from build123d import *

# Parameters (mm, degrees)
SKETCH1_R           = 9.5
BOSS_EXTRUDE1_DEPTH = 35
CUT_EXTRUDE1_DEPTH  = 4


with BuildPart() as part:
    # Sketch1 → Boss-Extrude1 (new body)
    with BuildSketch(Plane.XY):
        Circle(SKETCH1_R)
    extrude(amount=BOSS_EXTRUDE1_DEPTH)

    # Sketch4 → Cut-Extrude1 (cut)
    with BuildSketch(Plane(origin=(0, 10, 0), x_dir=(1, 0, 0), z_dir=(0, 1, 0))):
        with BuildLine():
            Line((3, 0), (3, -25))
            ThreePointArc((3, -25), (0, -28), (-3, -25))
            Line((-3, -25), (-3, 0))
            Line((-3, 0), (3, 0))
        make_face()
    extrude(amount=-CUT_EXTRUDE1_DEPTH, mode=Mode.SUBTRACT)


solid = part.part
Source: CAD feature listing. Evaluate the final solid. Frame: model axes, mm. A direction names the side the tool comes from. Give positions to 0.01 mm unless a question says otherwise; leave off trailing zeros. Write each loop counter-clockwise with the first axis right and the second up, starting at its lowest first coordinate (ties: lowest second). Pieces come first, ordered by that corner, then holes. Notation, with made-up numbers: M 73,-5.5 L 104,-5.5 A11 cw 104,4.5 Z; hole C 3,15 d7. An arc over 180 degrees is marked long. Return JSON: item names as keys, results as strings. Group by question number.
1) Set-up query: faces 1 (the face through (-3, 8, 13)), 2 (the face through (0, 0, 35)). Return all of +Z, -Z, +X, -X, +Y, -Y with unobstructed straight access to the full face (end or side cutting, diameter ignored); none if empty.
2) Cut plane A-A, the plane x = 0. Output: boundary loops of the cut face in (y, z), then the cut area to 3 significant figures.
3) Cut plane C-C, the plane y = -2.5. Output: boundary loops of the cut face in (x, z).
4) Ray query, L1, parallel to Y at x = -0.25, z = 30.5; L2, parallel to Y at x = 7, z = 17.5; L3, parallel to X at y = -2.75, z = 15.5. Return the intervals inside material, ascending.
5) Cut plane B-B, the plane z = 19.5. Output: boundary loops of the cut face in (x, y).
6) First-contact query: pin 1 Ø3 at (x, z) = (1, 12.5) entering from +Y; pin 2 Ø2 at (y, z) = (-3, 23) entering from -X; pin 3 Ø1.5 at (y, z) = (0.5, 8) entering from -X; pin 4 Ø2.5 at (y, z) = (7.5, 18.5) entering from -X. Flat tips, straight axial feed; report the tip coordinate or a pass-through.
7) Cut plane D-D, the plane x = 2.5. Output: boundary loops of the cut face in (y, z), then the cut area to 3 significant figures.
Data:
{
 "1": {"face 1": "-Z, +Y", "face 2": "+Z, +X, -X, +Y, -Y"},
 "2": {"outline": "M -9.5,0 L 6,0 L 6,28 L 9.5,28 L 9.5,35 L -9.5,35 Z", "area": "567 mm²"},
 "3": {"outline": "M -9.17,0 L 9.17,0 L 9.17,35 L -9.17,35 Z"},
 "4": {"L1": "y = -9.5 to 9.5", "L2": "y = -6.42 to 6.42", "L3": "x = -9.09 to 9.09"},
 "5": {"outline": "M -3,6 L -3,9.01 A9.5 ccw long 3,9.01 L 3,6 Z"},
 "6": {"pin 1": "stops at y = 6", "pin 2": "stops at x = -9.29", "pin 3": "stops at x = -9.5", "pin 4": "stops at x = -7.15"},
 "7": {"outline": "M -9.17,0 L 6,0 L 6,26.66 L 9.17,26.66 L 9.17,35 L -9.17,35 Z", "area": "557 mm²"}
}
